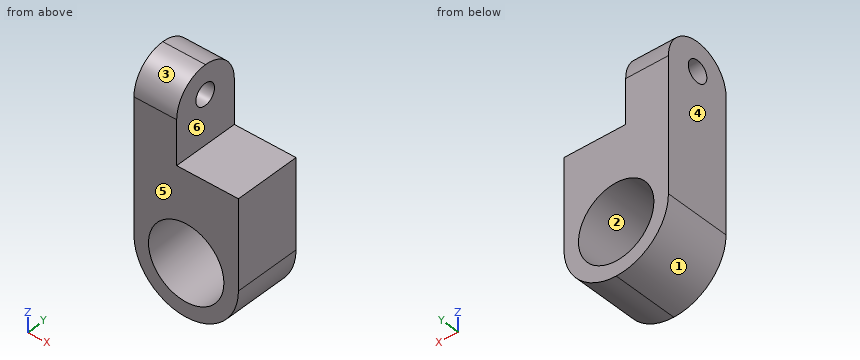
```python
from build123d import *

# Parameters (mm, degrees)
SKETCH1_W             = 23
SKETCH1_H             = 7
BOSS_EXTRUDE1_DEPTH   = 5.5
SKETCH2_R             = 3.96875
CUT_EXTRUDE1_DEPTH    = 15.543039572
SKETCH3_W             = 8.15
SKETCH3_H             = 7
CUT_EXTRUDE2_DEPTH    = 6.5
F_4_40_TAPPED_HOLE1_D = 2.2606
FILLET1_R             = 3.5
FILLET2_R             = 5.5


with BuildPart() as part:
    # Sketch1 → Boss-Extrude1 (new, symmetric)
    with BuildSketch(Plane(origin=(0, 0, 0), x_dir=(0, 0, -1), z_dir=(1, 0, 0))):
        Rectangle(SKETCH1_W, SKETCH1_H)
    extrude(amount=BOSS_EXTRUDE1_DEPTH, both=True)

    # Sketch2 → Cut-Extrude1 (cut, through all)
    with BuildSketch(Plane(origin=(0, 3.5, 0), x_dir=(1, 0, 0), z_dir=(0, 1, 0))):
        with Locations(Location((0, 6, 0), (0, 0, 270))):
            Circle(SKETCH2_R)
    extrude(amount=-CUT_EXTRUDE1_DEPTH, mode=Mode.SUBTRACT)

    # Sketch3 → Cut-Extrude2 (cut)
    with BuildSketch(Plane(origin=(5.5, 0, 0), x_dir=(0, 0, -1), z_dir=(1, 0, 0))):
        with Locations((-7.425, 0)):
            Rectangle(SKETCH3_W, SKETCH3_H)
    extrude(amount=-CUT_EXTRUDE2_DEPTH, mode=Mode.SUBTRACT)

    # #4-40 Tapped Hole1 (through all)
    with Locations(Plane(origin=(-1, 0, 0), x_dir=(0, 0, -1), z_dir=(1, 0, 0))):
        with Locations((-8.5, -0.04)):
            Hole(F_4_40_TAPPED_HOLE1_D / 2)

    # Fillet1
    fillet1_edges = [part.edges().sort_by_distance(p)[0] for p in [
        (-3.25, -3.5, 11.5),
        (-3.25, 3.5, 11.5),
    ]]
    fillet(fillet1_edges, radius=FILLET1_R - 0.0001)  # a hair under: the kernel refuses the full size

    # Fillet2
    fillet2_edges = [part.edges().sort_by_distance(p)[0] for p in [
        (-5.5, 0, -11.5),
        (5.5, 0, -11.5),
    ]]
    fillet(fillet2_edges, radius=FILLET2_R - 0.0001)  # a hair under: the kernel refuses the full size


solid = part.part
```
The model under review builds one solid part; all positions refer to its coordinate system, in mm. Face numbers are marked on the shaded views. A direction names the side the tool comes from. Round coordinates to 2 decimals unless told otherwise and drop trailing zeros. Loops run counter-clockwise (first coordinate to the right, second up) from the corner with the lowest first, then second, coordinate; pieces in that order, holes last. Notation, with made-up numbers: M -20.5,10.25 L -13.5,10.25 A20 ccw -13.5,37.25 Z; hole C 50.5,-11.75 d2. An arc over 180 degrees is marked long. Put each result on its own line as item: value.
Q1. Consider section D-D, the plane x = 2.25. Give the boundary of the cut face in (y, z), then the cut area to 3 significant figures.
Result set:
outline: M -3.5,-11.02 L 3.5,-11.02 L 3.5,-9.27 L -3.5,-9.27 Z; M -3.5,-2.73 L 3.5,-2.73 L 3.5,3.35 L -3.5,3.35 Z
area: 54.8 mm²
Q2. For pin 1 (3 mm diameter, centred on x = 3, y = 0.5, fed in from +Z); pin 2 (2 mm diameter, centred on y = 2.5, z = 5, fed in from +X); pin 3 (3 mm diameter, centred on y = -2.5, z = -9, fed in from +X), all flat-tipped, find the tip position at first contact; note any pin that passes through.
Result set:
pin 1: stops at z = 3.35
pin 2: stops at x = -1
pin 3: stops at x = 5.29
Q3. Mouldability with a two-part tool opening along Z and no side actions: class the marked faces 1, 2, 3 and 4 as released by +Z, released by -Z, zero draft, split by the parting line, or undercut.
Result set:
face 1: released by -Z
face 2: undercut
face 3: released by +Z
face 4: zero draft
Q4. Consider section A-A, the plane y = 0.5. Count the separate pieces of the cut face and the enclosed holes in it, then the cut area to 3 significant figures.
Result set:
separate pieces: 2
enclosed holes: 1
area: 128 mm²
Q5. To check wall thickness, follow L1, parallel to Z at x = -1.5, y = -1; L2, parallel to X at y = -1, z = -6; L3, parallel to Z at x = -3.5, y = -0.25. State the ranges of each line that lie inside material, in increasing order.
Result set:
L1: z = -11.29 to -9.67, -2.33 to 7.9, 9.1 to 11.35
L2: x = -5.5 to -3.97, 3.97 to 5.5
L3: z = -10.24 to -7.87, -4.13 to 7.39, 9.61 to 11.49
Q6. Machinability: for the marked faces 5 and 6, which of the approach directions +Z, -Z, +X, -X, +Y, -Y give a long, thin tool a straight path to every point of the face, cutting with its end or side? Answer none if there is none.
Result set:
face 5: +Z, -Z, +X, -X, -Y
face 6: +Z, +X, +Y, -Y
Q7. Consider section C-C, the plane z = -9.5. Give the boundary of the cut face in (x, y), then the cut area to 3 significant figures.
Result set:
outline: M -4.24,-3.5 L -1.87,-3.5 L -1.87,3.5 L -4.24,3.5 Z; M 1.87,-3.5 L 4.24,-3.5 L 4.24,3.5 L 1.87,3.5 Z
area: 33.2 mm²
